Work out the finished part from the listing and answer in its coordinate system (mm). Face numbers are marked on the shaded views. A direction names the side the tool comes from. Round coordinates to 2 decimals unless told otherwise and drop trailing zeros. Order: outer loops, then holes, each group sorted by start corner. A loop starts at its lowest first (then second) coordinate and runs counter-clockwise, first axis right, second up. Notation, with made-up numbers: M 34.25,12 L 71.25,12 A14 cw 71.25,18 Z; hole C 81,49.25 d7. An arc over 180 degrees is marked long. Return JSON: item names as keys, results as strings.
from build123d import *

# Parameters (mm, degrees)
SKETCH1_W             = 12.7
SKETCH1_H             = 88.9
BOSS_EXTRUDE1_DEPTH   = 63.5
BOSS_EXTRUDE1_2_DEPTH = 63.5
BOSS_EXTRUDE2_DEPTH   = 12.7
SKETCH3_W             = 114.3
SKETCH3_H             = 12.7
CUT_EXTRUDE1_DEPTH    = 208.03236895


with BuildPart() as part:
    # Sketch1 → Boss-Extrude1 (new body)
    with BuildSketch(Plane(origin=(0, 0, 0), x_dir=(1, 0, 0), z_dir=(0, 1, 0))):
        with Locations((6.35, 44.45)):
            Rectangle(SKETCH1_W, SKETCH1_H)
    extrude(amount=BOSS_EXTRUDE1_DEPTH)



with BuildPart() as body_2:
    # Sketch1 → Boss-Extrude1 2 (new body)
    with BuildSketch(Plane(origin=(0, 0, 0), x_dir=(1, 0, 0), z_dir=(0, 1, 0))):
        with Locations((-133.35, 44.45)):
            Rectangle(SKETCH1_W, SKETCH1_H)
    extrude(amount=BOSS_EXTRUDE1_2_DEPTH)


with BuildPart() as part_1:
    add(part.part)

    add(body_2.part)  # Boss-Extrude2 merges body 2
    # Sketch2 → Boss-Extrude2 (add)
    with BuildSketch(Plane(origin=(0, 63.5, 0), x_dir=(1, 0, 0), z_dir=(0, 1, 0))):
        Polygon((-63.5, -43.538181024), (12.7, 0.455909488), (12.7, 88.444090512), (-63.5, 132.438181024), (-139.7, 88.444090512), (-139.7, 0.455909488), align=None)
    extrude(amount=BOSS_EXTRUDE2_DEPTH)

    # Sketch3 → Cut-Extrude1 (cut, through all)
    with BuildSketch(Plane(origin=(0, 76.2, 0), x_dir=(1, 0, 0), z_dir=(0, 1, 0))):
        with Locations((-63.5, 6.805909488)):
            Rectangle(SKETCH3_W, SKETCH3_H)
        with Locations((-63.5, 82.094090512)):
            Rectangle(SKETCH3_W, SKETCH3_H)
    extrude(amount=-CUT_EXTRUDE1_DEPTH, mode=Mode.SUBTRACT)


solid = part_1.part
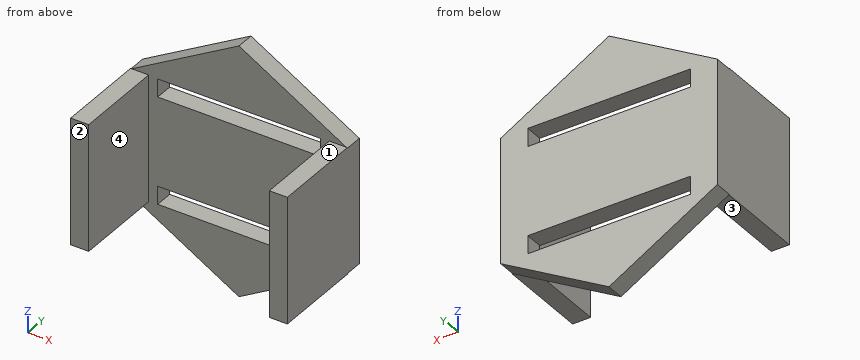
Item 1: Find section C-C (z = -19). Determine the outline of the cut face in (x, y), plus the area to 3 significant figures.
Output:
{"outline": "M -139.7,0 L -127,0 L -127,63.5 L 0,63.5 L 0,0 L 12.7,0 L 12.7,76.2 L -139.7,76.2 Z", "area": "3,550 mm^2"}
Item 2: Each of these flat-tipped pins is pushed along its axis until it touches: pin 1 (6.5 mm diameter, centred on x = -72.5, y = 67.5, fed in from +Z); pin 2 (0.5 mm diameter, centred on x = 12.5, z = 0, fed in from +Y); pin 3 (10 mm diameter, centred on x = -73, y = 71, fed in from -Z); pin 4 (10 mm diameter, centred on x = -62, y = 68.5, fed in from -Z). Where does it stop, or does it pass through?
Output:
{"pin 1": "stops at z = 40.22", "pin 2": "stops at y = 63.5", "pin 3": "stops at z = -129.84", "pin 4": "stops at z = -132.44"}
Item 3: Consider line 1 along X through (y, z) = (36, -55.5); line 2 along Z through (x, y) = (-16.5, 64.5); line 3 along Y through (x, z) = (-59.5, 15). Determine where each line is inside the solid, lowest interval first. Write a range as [from, to].
Output:
{"line 1": "x = [-139.7, -127], [0, 12.7]", "line 2": "z = [-105.3, -88.44], [-75.74, -13.16], [-0.46, 16.4]", "line 3": "y = [63.5, 76.2]"}
Item 4: Find section A-A (y = 41). Determine the outline of the cut face in (x, z), plus the area to 3 significant figures.
Output:
{"outline": "M -139.7,-88.9 L -127,-88.9 L -127,0 L -139.7,0 Z; M 0,-88.9 L 12.7,-88.9 L 12.7,0 L 0,0 Z", "area": "2,260 mm^2"}
Item 5: Find section B-B (x = -38.5). Determine the outline of the cut face in (y, z).
Output:
{"outline": "M 63.5,-118 L 76.2,-118 L 76.2,-88.44 L 63.5,-88.44 Z; M 63.5,-75.74 L 76.2,-75.74 L 76.2,-13.16 L 63.5,-13.16 Z; M 63.5,-0.46 L 76.2,-0.46 L 76.2,29.1 L 63.5,29.1 Z"}
Item 6: Which of the six approach directions +Z, -Z, +X, -X, +Y, -Y give full straight-line access (tool end or side, diameter ignored) to the marked faces 1, 2, 3 and 4?
Output:
{"face 1": "+Z, +X, -X, -Y", "face 2": "+Z, -Z, +X, -X, -Y", "face 3": "-Z, +X, -X, -Y", "face 4": "+Z, -Z, -Y"}
Item 7: Find section D-D (x = -98.5). Determine the outline of the cut face in (y, z), plus the area to 3 significant figures.
Output:
{"outline": "M 63.5,-112.23 L 76.2,-112.23 L 76.2,-88.44 L 63.5,-88.44 Z; M 63.5,-75.74 L 76.2,-75.74 L 76.2,-13.16 L 63.5,-13.16 Z; M 63.5,-0.46 L 76.2,-0.46 L 76.2,23.33 L 63.5,23.33 Z", "area": "1,400 mm^2"}
